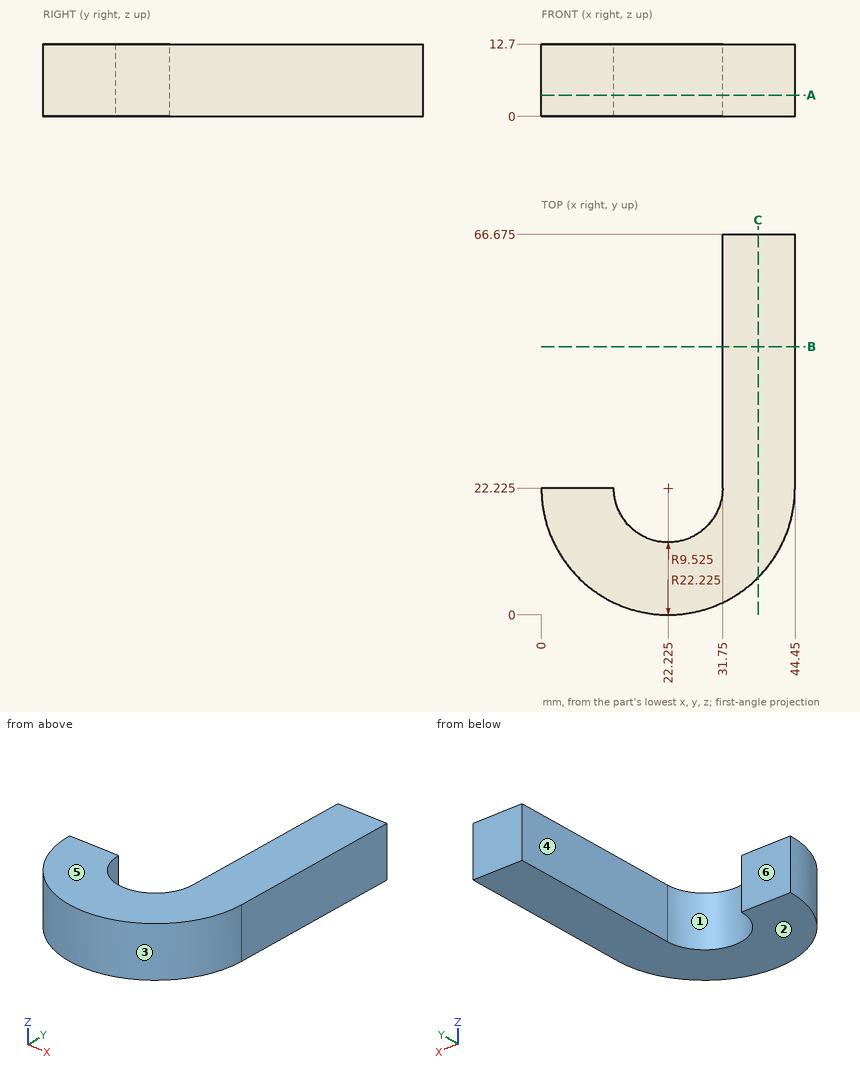
Input: dimensioned drawing with shaded views. Units: mm. Origin: part minimum x, y, z. A direction names the side the tool comes from. Give positions to 0.01 mm unless a question says otherwise; leave off trailing zeros. Write each loop counter-clockwise with the first axis right and the second up, starting at its lowest first coordinate (ties: lowest second). Pieces come first, ordered by that corner, then holes.
1. Section query C-C (x = 38). Return the cut outline in (y, z) (3 decimals).
2. Section query B-B (y = 47). Return the cut outline in (x, z).
3. Pull-direction query (X, two-part tool) for the marked faces 1, 2, 3 and 4; classes: +X half, -X half, draft (parallel to the pull), parting line (faces both ways), or undercut.
4. Access query for the marked faces 5 and 6. Directions: +Z, -Z, +X, -X, +Y, -Y. A direction counts if a zero-diameter tool reaches every point of the face in a straight line with its end or side. Return the directions, or none.
5. Section query A-A (z = 3.75). Return the cut outline in (x, y) (3 decimals).
6. Material intervals for line 1 along X through (y, z) = (27, 11.75); line 2 along Y through (x, z) = (22, 3.25); line 3 along X through (y, z) = (21.5, 7.75), sorted ascending.
7. First-contact query: pin 1 (4 mm diameter, centred on x = 37, z = 7, fed in from -Y); pin 2 (5 mm diameter, centred on x = 27.5, z = 2, fed in from -Y); pin 3 (1.5 mm diameter, centred on x = 10.5, z = 6.5, fed in from -Y). Flat tips, straight axial feed; report the tip coordinate or a pass-through.
Output values:
1. outline: (6.569, 0) - (66.675, 0) - (66.675, 12.7) - (6.569, 12.7) - close
2. outline: (31.75, 0) - (44.45, 0) - (44.45, 12.7) - (31.75, 12.7) - close
3. face 1: undercut
3. face 2: draft
3. face 3: parting line
3. face 4: -X half
4. face 5: +Z, +X, -X, +Y, -Y
4. face 6: +Z, -Z, -X, +Y
5. outline: (0, 22.225) arc R22.225 ccw to (44.45, 22.225) - (44.45, 66.675) - (31.75, 66.675) - (31.75, 22.225) arc R9.525 cw to (12.7, 22.225) - close
6. line 1: x = 31.75 to 44.45
6. line 2: y = 0 to 12.7
6. line 3: x = 0.01 to 12.73, 31.72 to 44.44
7. pin 1: stops at y = 4.04
7. pin 2: stops at y = 0.17
7. pin 3: stops at y = 2.9
